Build history of the part. All positions in model axes, mm. Face numbers are marked on the shaded views. A direction names the side the tool comes from. Round coordinates to 2 decimals unless told otherwise and drop trailing zeros. Order: outer loops, then holes, each group sorted by start corner. A loop starts at its lowest first (then second) coordinate and runs counter-clockwise, first axis right, second up. Notation, with made-up numbers: M 36.5,-34 L 69.5,-34 A30 cw 69.5,-3 Z; hole C -16.75,86.5 d11. An arc over 180 degrees is marked long. One line per item, written item: value. Start each with the question number.
Item 1: Tool access for the marked faces 4, 5, 6, 7 and 8: list every direction of +Z, -Z, +X, -X, +Y, -Y with a clear straight run to the whole face (end or side of a thin tool).
Item 2: Band-saw the part on D-D, the plane z = 0. Write the cut outline in (x, y).
Item 3: Band-saw the part on A-A, the plane z = -8.5. Write the cut outline in (x, y), then the cut area to 3 significant figures.
Item 4: Band-saw the part on C-C, the plane x = 10.75. Write the cut outline in (y, z), then the cut area to 3 significant figures.
Item 5: Band-saw the part on B-B, the plane y = 10. Write the cut outline in (x, z).
Item 6: Probe L1, parallel to X at y = 4, z = 9.75; L2, parallel to X at y = 7, z = 6; L3, parallel to X at y = 11, z = 7.25. List the from-to ranges inside material, lowest first.
Item 7: Pin check, flat tips, straight feed: pin 1 (4 mm diameter, centred on y = 9, z = 1.5, fed in from -X); pin 2 (1.2 mm diameter, centred on x = 5, z = -0.5, fed in from -Y). Stop position of each tip, or through.
Item 8: Two-plate mould, pull along X, no slides. Class the marked faces 1, 2 and 3: +X half, -X half, draft (parallel to the pull), parting line (faces both ways), or undercut.
```python
from build123d import *

# Parameters (mm, degrees)
SKETCH1_W           = 27.5
SKETCH1_H           = 21
BOSS_EXTRUDE1_DEPTH = 12
SKETCH4_W           = 4
SKETCH4_H           = 2
CUT_EXTRUDE1_DEPTH  = 28.821978722
FILLET1_R           = 5


with BuildPart() as part:
    # Sketch1 → Boss-Extrude1 (new body)
    with BuildSketch(Plane(origin=(0, 0, 0), x_dir=(1, 0, 0), z_dir=(0, 1, 0))):
        Rectangle(SKETCH1_W, SKETCH1_H)
    extrude(amount=BOSS_EXTRUDE1_DEPTH)

    # Sketch2 → Cut-Revolve1 (revolve, cut)
    with BuildSketch(Plane(origin=(0, 12, 0), x_dir=(1, 0, 0), z_dir=(0, 1, 0))):
        Polygon((-13.75, 0), (13.75, 0), (13.75, 4.5), (11.25, 4.5), (11.25, 8), (7, 8), (7, 7.6), (6, 7.6), (6, 8), (-8.5, 8), (-8.5, 7.6), (-9.5, 7.6), (-9.5, 8), (-13.75, 8), align=None)
    revolve(axis=Axis((-13.75, 12, 0), (1, 0, 0)), mode=Mode.SUBTRACT)

    # Sketch4 → Cut-Extrude1 (cut, through all)
    with BuildSketch(Plane.XY.offset(10.5)):
        with Locations((-8.25, 1)):
            Rectangle(SKETCH4_W, SKETCH4_H)
        with Locations((5.75, 1)):
            Rectangle(SKETCH4_W, SKETCH4_H)
    extrude(amount=-CUT_EXTRUDE1_DEPTH, mode=Mode.SUBTRACT)

    # Fillet1
    fillet1_edges = [part.edges().sort_by_distance(p)[0] for p in [
        (-8.25, 2, -10.5),
        (-8.25, 2, 10.5),
        (5.75, 2, -10.5),
        (5.75, 2, 10.5),
    ]]
    fillet(fillet1_edges, radius=FILLET1_R)


solid = part.part
```
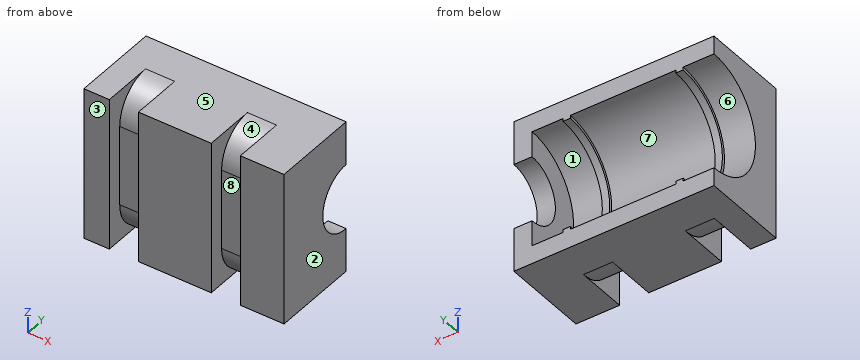
Output:
1. face 4: +Z, -Y
1. face 5: +Z, +X, -X, +Y, -Y
1. face 6: -X, +Y
1. face 7: +Y
1. face 8: +Z, -Z, -Y
2. outline: M -13.75,0 L -10.25,0 L -10.25,2 L -6.25,2 L -6.25,0 L 3.75,0 L 3.75,2 L 7.75,2 L 7.75,0 L 13.75,0 L 13.75,7.5 L 11.25,7.5 L 11.25,4 L 7,4 L 7,4.4 L 6,4.4 L 6,4 L -8.5,4 L -8.5,4.4 L -9.5,4.4 L -9.5,4 L -13.75,4 Z
3. outline: M -13.75,0 L -10.25,0 L -10.25,3 L -6.25,3 L -6.25,0 L 3.75,0 L 3.75,3 L 7.75,3 L 7.75,0 L 13.75,0 L 13.75,12 L -13.75,12 Z
3. area: 306 mm²
4. outline: M 0,-10.5 L 12,-10.5 L 12,-8 A8 cw 12,8 L 12,10.5 L 0,10.5 Z
4. area: 151 mm²
5. outline: M -13.75,-10.5 L 13.75,-10.5 L 13.75,-4.03 L 11.25,-4.03 L 11.25,-7.75 L 7,-7.75 L 7,-7.33 L 6,-7.33 L 6,-7.75 L -8.5,-7.75 L -8.5,-7.33 L -9.5,-7.33 L -9.5,-7.75 L -13.75,-7.75 Z; M -13.75,7.75 L -9.5,7.75 L -9.5,7.33 L -8.5,7.33 L -8.5,7.75 L 6,7.75 L 6,7.33 L 7,7.33 L 7,7.75 L 11.25,7.75 L 11.25,4.03 L 13.75,4.03 L 13.75,10.5 L -13.75,10.5 Z
6. L1: x = -13.75 to -10.25, -6.25 to 3.75, 7.75 to 13.75
6. L2: x = -9.5 to -8.5, 6 to 7, 11.25 to 13.75
6. L3: x = 11.25 to 13.75
7. pin 1: stops at x = 11.25
7. pin 2: stops at y = 2
8. face 1: undercut
8. face 2: +X half
8. face 3: draft
